```python
from build123d import *

# Parameters (mm, degrees)
SKETCH_1_R          = 2.5
EXTRUDE_1_DEPTH     = 3
FILLET_1_R          = 0.5
CUT_EXTRUDE_1_DEPTH = 2
SKETCH_3_R          = 1.5
EXTRUDE_2_DEPTH     = 6
CHAMFER_1_SIZE      = 0.2
FILLET_2_R          = 0.2


with BuildPart() as part:
    # 草图1 → 凸台-拉伸1 (new body)
    with BuildSketch(Plane.XY):
        Circle(SKETCH_1_R)
    extrude(amount=EXTRUDE_1_DEPTH)

    # 圆角1
    fillet_1_edges = [part.edges().sort_by_distance(p)[0] for p in [
        (-2.5, 0, 3),
    ]]
    fillet(fillet_1_edges, radius=FILLET_1_R)

    # 草图2 → 切除-拉伸1 (cut)
    with BuildSketch(Plane.XY.offset(3)):
        Polygon((1.558845727, 0), (0.779422863, 1.35), (-0.779422863, 1.35), (-1.558845727, 0), (-0.779422863, -1.35), (0.779422863, -1.35), align=None)
    extrude(amount=-CUT_EXTRUDE_1_DEPTH, mode=Mode.SUBTRACT)

    # 草图3 → 凸台-拉伸2 (add)
    with BuildSketch(Plane(origin=(0, 0, 0), x_dir=(-1, 0, 0), z_dir=(0, 0, -1))):
        Circle(SKETCH_3_R)
    extrude(amount=EXTRUDE_2_DEPTH)

    # 倒角1
    chamfer_1_edges = [part.edges().sort_by_distance(p)[0] for p in [
        (1.5, 0, -6),
    ]]
    chamfer(chamfer_1_edges, length=CHAMFER_1_SIZE)

    # 圆角2
    fillet_2_edges = [part.edges().sort_by_distance(p)[0] for p in [
        (-2.5, 0, 0),
    ]]
    fillet(fillet_2_edges, radius=FILLET_2_R)


solid = part.part
```
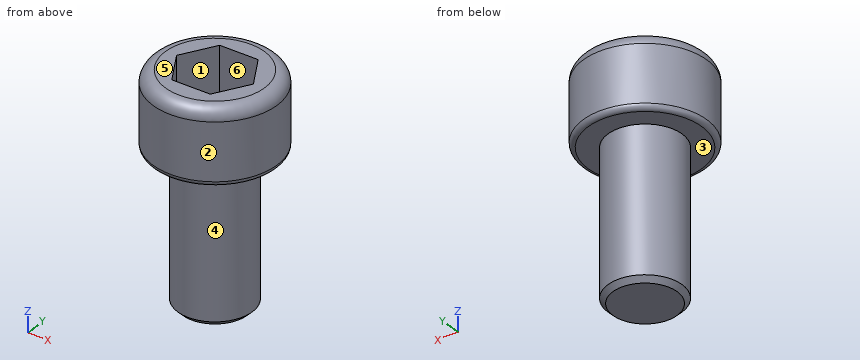
The listing builds one solid part. Answer for the finished solid, in the listing's coordinates (mm). Face numbers are marked on the shaded views. A direction names the side the tool comes from. Round coordinates to 2 decimals unless told otherwise and drop trailing zeros. Loops run counter-clockwise (first coordinate to the right, second up) from the corner with the lowest first, then second, coordinate; pieces in that order, holes last. Notation, with made-up numbers: (42, 27) - (100, 27) arc R27 cw to (100, 50) - close; hole circle Ø9 at (0.5, 53.5). An arc over 180 degrees is marked (long way). Return JSON: item names as keys, results as strings. Group by question number.
1. The part is cut by section C-C on z = 0.75. Determine the outline of the cut face in (x, y), then the cut area to 3 significant figures.
2. The part is cut by section D-D on z = -5.25. Determine the outline of the cut face in (x, y), then the cut area to 3 significant figures.
3. Which of the six approach directions +Z, -Z, +X, -X, +Y, -Y give full straight-line access (tool end or side, diameter ignored) to the marked faces 1, 2 and 3?
4. The mould has two halves that part along Y. Classify the marked faces 4, 5 and 6: pulls with the +Y half, pulls with the -Y half, needs draft (parallel to the pull), parting line crosses it, or undercut.
5. This flat-tipped pin is pushed along its axis until it touches: P1, Ø0.8, axis at x = 0, y = 0, coming from the +Z side. Where does it stop, or does it pass through?
6. The part is cut by section B-B on x = 0. Determine the outline of the cut face in (y, z), then the cut area to 3 significant figures.
7. The part is cut by section A-A on z = 1.75. Determine the outline of the cut face in (x, y), then the cut area to 3 significant figures.
8. Consider probe 1 along Z at (x, y) = (0, 1.8); probe 2 along X at (y, z) = (-0.45, 1.25); probe 3 along X at (y, z) = (-1.3, 1.5). Determine where each line is inside the solid, lowest interval first.
Resolved:
{
 "1": {"outline": "circle Ø5 at (0, 0)", "area": "19.6 mm²"},
 "2": {"outline": "circle Ø3 at (0, 0)", "area": "7.07 mm²"},
 "3": {"face 1": "+Z", "face 2": "+Z, -Z", "face 3": "-Z"},
 "4": {"face 4": "parting line crosses it", "face 5": "needs draft", "face 6": "undercut"},
 "5": {"P1": "stops at z = 1"},
 "6": {"outline": "(-2.5, 0.2) arc R0.2 ccw to (-2.3, 0) - (-1.5, 0) - (-1.5, -5.8) - (-1.3, -6) - (1.3, -6) - (1.5, -5.8) - (1.5, 0) - (2.3, 0) arc R0.2 ccw to (2.5, 0.2) - (2.5, 2.5) arc R0.5 ccw to (2, 3) - (1.35, 3) - (1.35, 1) - (-1.35, 1) - (-1.35, 3) - (-2, 3) arc R0.5 ccw to (-2.5, 2.5) - close", "area": "27.4 mm²"},
 "7": {"outline": "circle Ø5 at (0, 0); hole (-1.56, 0) - (-0.78, -1.35) - (0.78, -1.35) - (1.56, 0) - (0.78, 1.35) - (-0.78, 1.35) - close", "area": "13.3 mm²"},
 "8": {"probe 1": "z = 0 to 3", "probe 2": "x = -2.46 to -1.3, 1.3 to 2.46", "probe 3": "x = -2.14 to -0.81, 0.81 to 2.14"}
}
